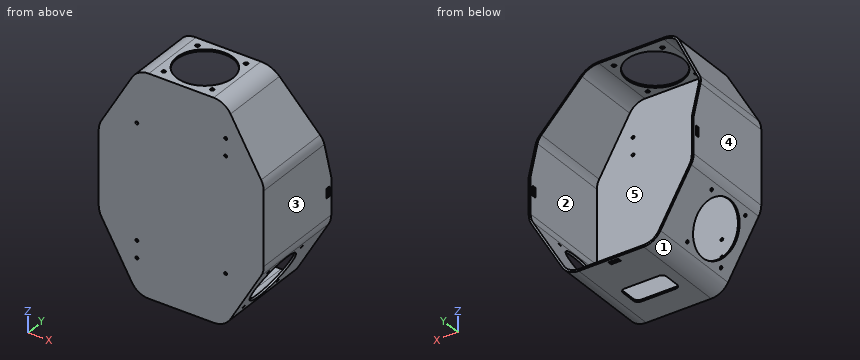
```python
from build123d import *

# Parameters (mm, degrees)
SALIENTE_EXTRUIR1_DEPTH     = 100
VACIADO2_T                  = -2
CROQUIS2_R                  = 1.5
CORTAR_EXTRUIR1_DEPTH       = 101
CORTAR_EXTRUIR1_DEPTH_BACK  = 1
CROQUIS8_R                  = 28
CROQUIS8_R_2                = 1.5
CORTAR_EXTRUIR6_DEPTH       = 130.862159322
CORTAR_EXTRUIR7_DEPTH       = 113.5
CORTAR_EXTRUIR8_DEPTH       = 86
CORTAR_EXTRUIR8_DEPTH_BACK  = 86
CROQUIS11_R                 = 29
CROQUIS11_R_2               = 2
CORTAR_EXTRUIR9_DEPTH       = 113.5
CROQUIS13_W                 = 10
CROQUIS13_H                 = 4
CORTAR_EXTRUIR10_DEPTH      = 113.5
CROQUIS14_W                 = 10
CROQUIS14_H                 = 4
CORTAR_EXTRUIR11_DEPTH      = 86
CORTAR_EXTRUIR11_DEPTH_BACK = 86


with BuildPart() as part:
    # Croquis1 → Saliente-Extruir1 (new body)
    with BuildSketch(Plane(origin=(0, 0, 0), x_dir=(1, 0, 0), z_dir=(0, 1, 0))):
        with BuildLine():
            Line((-82.320508076, 47.858983849), (-50.773502692, 102.5))
            ThreePointArc((-50.773502692, 102.5), (-43.452994616, 109.820508076), (-33.452994616, 112.5))
            Line((-33.452994616, 112.5), (33.452994616, 112.5))
            ThreePointArc((33.452994616, 112.5), (43.452994616, 109.820508076), (50.773502692, 102.5))
            Line((50.773502692, 102.5), (82.320508076, 47.858983849))
            ThreePointArc((82.320508076, 47.858983849), (84.318516526, 43.035364751), (85, 37.858983849))
            Line((85, 37.858983849), (85, -37.858983849))
            ThreePointArc((85, -37.858983849), (84.318516526, -43.035364751), (82.320508076, -47.858983849))
            Line((82.320508076, -47.858983849), (50.773502692, -102.5))
            ThreePointArc((50.773502692, -102.5), (43.452994616, -109.820508076), (33.452994616, -112.5))
            Line((33.452994616, -112.5), (-33.452994616, -112.5))
            ThreePointArc((-33.452994616, -112.5), (-43.452994616, -109.820508076), (-50.773502692, -102.5))
            Line((-50.773502692, -102.5), (-82.320508076, -47.858983849))
            ThreePointArc((-82.320508076, -47.858983849), (-84.318516526, -43.035364751), (-85, -37.858983849))
            Line((-85, -37.858983849), (-85, 37.858983849))
            ThreePointArc((-85, 37.858983849), (-84.318516526, 43.035364751), (-82.320508076, 47.858983849))
        make_face()
    extrude(amount=SALIENTE_EXTRUIR1_DEPTH)

    # Vaciado2
    vaciado2_openings = [part.faces().sort_by_distance(p)[0] for p in [
        (0, 100, 0),
    ]]
    offset(amount=VACIADO2_T, openings=vaciado2_openings, kind=Kind.INTERSECTION)

    # Croquis2 → Cortar-Extruir1 (cut, two sides)
    with BuildSketch(Plane(origin=(0, 0, 0), x_dir=(1, 0, 0), z_dir=(0, 1, 0))) as cortar_extruir1_sk:
        with Locations((-45.75, 76.25)):
            Circle(CROQUIS2_R)
        with Locations((-45.75, 58.75)):
            Circle(CROQUIS2_R)
        with Locations((45.75, 58.75)):
            Circle(CROQUIS2_R)
        with Locations((-45.75, -58.75)):
            Circle(CROQUIS2_R)
        with Locations((45.75, -58.75)):
            Circle(CROQUIS2_R)
        with Locations((45.75, -76.25)):
            Circle(CROQUIS2_R)
    extrude(amount=CORTAR_EXTRUIR1_DEPTH, mode=Mode.SUBTRACT)
    extrude(cortar_extruir1_sk.sketch, amount=-CORTAR_EXTRUIR1_DEPTH_BACK, mode=Mode.SUBTRACT)

    # Croquis8 → Cortar-Extruir6 (cut, through all)
    with BuildSketch(Plane(origin=(0, 0, 0), x_dir=(-0.5, 0, -0.866025404), z_dir=(0.866025404, 0, -0.5))):
        with Locations((31.833847158, 40)):
            Circle(CROQUIS8_R)
        with Locations((6.833847158, 65)):
            Circle(CROQUIS8_R_2)
        with Locations((56.833847158, 65)):
            Circle(CROQUIS8_R_2)
        with Locations((6.833847158, 15)):
            Circle(CROQUIS8_R_2)
        with Locations((56.833847158, 15)):
            Circle(CROQUIS8_R_2)
    cortar_extruir6 = extrude(amount=CORTAR_EXTRUIR6_DEPTH, mode=Mode.SUBTRACT)

    # Simetría1: Cortar-Extruir6 across plane
    add(cortar_extruir6.mirror(Plane(origin=(0, 0, 0), x_dir=(0, 0, 1), z_dir=(1, 0, 0))), mode=Mode.SUBTRACT)

    # Croquis9 → Cortar-Extruir7 (cut, through all)
    with BuildSketch(Plane.XY):
        with BuildLine():
            Line((17.5, 55), (-17.5, 55))
            ThreePointArc((-17.5, 55), (-21.035533906, 53.535533906), (-22.5, 50))
            Line((-22.5, 50), (-22.5, 35))
            ThreePointArc((-22.5, 35), (-21.035533906, 31.464466094), (-17.5, 30))
            Line((-17.5, 30), (17.5, 30))
            ThreePointArc((17.5, 30), (21.035533906, 31.464466094), (22.5, 35))
            Line((22.5, 35), (22.5, 50))
            ThreePointArc((22.5, 50), (21.035533906, 53.535533906), (17.5, 55))
        make_face()
    extrude(amount=-CORTAR_EXTRUIR7_DEPTH, mode=Mode.SUBTRACT)

    # Croquis10 → Cortar-Extruir8 (cut, two sides)
    with BuildSketch(Plane(origin=(0, 0, 0), x_dir=(0, 0, -1), z_dir=(1, 0, 0))) as cortar_extruir8_sk:
        Polygon((0, 100), (-148.82762011, 60.12175938), (-148.82762011, 114.287226581), (0, 114.287226581), align=None)
    extrude(amount=CORTAR_EXTRUIR8_DEPTH, mode=Mode.SUBTRACT)
    extrude(cortar_extruir8_sk.sketch, amount=-CORTAR_EXTRUIR8_DEPTH_BACK, mode=Mode.SUBTRACT)

    # Croquis11 → Cortar-Extruir9 (cut, through all)
    with BuildSketch(Plane.XY):
        with Locations((0, 35)):
            Circle(CROQUIS11_R)
        with Locations((25, 10)):
            Circle(CROQUIS11_R_2)
        with Locations((-25, 10)):
            Circle(CROQUIS11_R_2)
        with Locations((-25, 60)):
            Circle(CROQUIS11_R_2)
        with Locations((25, 60)):
            Circle(CROQUIS11_R_2)
    extrude(amount=CORTAR_EXTRUIR9_DEPTH, mode=Mode.SUBTRACT)

    # Croquis13 → Cortar-Extruir10 (cut, through all)
    with BuildSketch(Plane.XY):
        with Locations((0, 95)):
            Rectangle(CROQUIS13_W, CROQUIS13_H)
    extrude(amount=-CORTAR_EXTRUIR10_DEPTH, mode=Mode.SUBTRACT)

    # Croquis14 → Cortar-Extruir11 (cut, two sides)
    with BuildSketch(Plane(origin=(0, 0, 0), x_dir=(0, 0, -1), z_dir=(1, 0, 0))) as cortar_extruir11_sk:
        with Locations((12.858983849, 95)):
            Rectangle(CROQUIS14_W, CROQUIS14_H)
    extrude(amount=CORTAR_EXTRUIR11_DEPTH, mode=Mode.SUBTRACT)
    extrude(cortar_extruir11_sk.sketch, amount=-CORTAR_EXTRUIR11_DEPTH_BACK, mode=Mode.SUBTRACT)


solid = part.part
```
Check sheet for the modelled part. Datum: model origin and axes. Units: mm. Face numbers are marked on the shaded views. A direction names the side the tool comes from. Give positions to 0.01 mm unless a question says otherwise; leave off trailing zeros. Order: outer loops, then holes, each group sorted by start corner. A loop starts at its lowest first (then second) coordinate and runs counter-clockwise, first axis right, second up. Notation, with made-up numbers: M 73.25,-4 L 106.25,-4 A34 cw 106.25,32 Z; hole C 53,-15 d7. An arc over 180 degrees is marked long. Answer in a Markdown table with one row per item.
1) Cross-section at B-B, the plane z = 71. Enter the section's corners in (x, y), plus the area to 3 significant figures.
Filled sheet:
| item | result |
|---|---|
| outline | M -68.96,0 L 68.96,0 L 68.96,80.98 L 66.65,80.98 L 66.65,2 L -66.65,2 L -66.65,80.98 L -68.96,80.98 Z |
| area | 641 mm2 |
2) Access from +Z, -Z, +X, -X, +Y, -Y to the whole of each face (thin tool, end or side, straight path). Record for the marked faces 4 and 5.
Filled sheet:
| item | result |
|---|---|
| face 4 | +Z, -Z, -X, +Y, -Y |
| face 5 | +Y |
3) Cross-section at A-A, the plane x = -15. Enter the section's corners in (y, z), plus the area to 3 significant figures.
Filled sheet:
| item | result |
|---|---|
| outline | M 0,-112.5 L 30,-112.5 L 30,-110.5 L 2,-110.5 L 2,110.5 L 10.18,110.5 L 10.18,112.5 L 0,112.5 Z; M 55,-112.5 L 100,-112.5 L 100,-110.5 L 55,-110.5 Z; M 59.82,110.5 L 70.39,110.5 L 69.86,112.5 L 59.82,112.5 Z |
| area | 633 mm2 |
4) Thickness scan on L1, parallel to X at y = 70, z = 9; L2, parallel to Z at x = 45.75, y = 1.5; L3, parallel to Z at x = 45, y = 1. Record the ranges inside material, lowest first. Write a range as [from, to].
Filled sheet:
| item | result |
|---|---|
| L1 | x = [-85, -83], [83, 85] |
| L2 | z = [-108.27, -60.25], [-57.25, 57.25], [60.25, 74.75], [77.75, 108.27] |
| L3 | z = [-108.83, -60.05], [-57.45, 57.45], [60.05, 74.95], [77.55, 108.83] |
5) Gauge pin test, flat ends, axial feed: P1, Ø1.8, axis at x = 45.75, z = -58.75, coming from the -Y side; P2, Ø1, axis at x = 61, z = 83.5, coming from the -Y side; P3, Ø8, axis at y = 76.5, z = 79, coming from the -X side; P4, Ø8, axis at y = 74.5, z = -47.5, coming from the -X side. Record the tip position at first contact, or that the pin passes through.
Filled sheet:
| item | result |
|---|---|
| P1 | passes through |
| P2 | stops at y = 0 |
| P3 | stops at x = -66.65 |
| P4 | stops at x = -84.19 |
6) Cross-section at C-C, the plane z = -66. Count the separate pieces of the cut face and the enclosed holes in it, plus the area to 3 significant figures.
Filled sheet:
| item | result |
|---|---|
| separate pieces | 3 |
| enclosed holes | 0 |
| area | 499 mm2 |
7) Release check for a two-part mould opening along X. For the marked faces 1, 2 and 3 record: +X half, -X half, draft (parallel to the pull), parting line (faces both ways), or undercut.
Filled sheet:
| item | result |
|---|---|
| face 1 | -X half |
| face 2 | undercut |
| face 3 | +X half |
